from build123d import *

# Parameters (mm, degrees)
SKETCH1_W           = 15
SKETCH1_H           = 30
SKETCH1_R           = 2.5
BOSS_EXTRUDE1_DEPTH = 3
SKETCH2_W           = 15
SKETCH2_H           = 18
SKETCH2_R           = 2.5
BOSS_EXTRUDE2_DEPTH = 3
BOSS_EXTRUDE3_DEPTH = 2


with BuildPart() as part:
    # Sketch1 → Boss-Extrude1 (new body)
    with BuildSketch(Plane.XY):
        Rectangle(SKETCH1_W, SKETCH1_H)
        with Locations((0, 8)):
            Circle(SKETCH1_R, mode=Mode.SUBTRACT)
        with Locations((0, -8)):
            Circle(SKETCH1_R, mode=Mode.SUBTRACT)
    extrude(amount=BOSS_EXTRUDE1_DEPTH)

    # Sketch2 → Boss-Extrude2 (add)
    with BuildSketch(Plane(origin=(0, 15, 0), x_dir=(1, 0, 0), z_dir=(0, 1, 0))):
        with Locations((0, 6)):
            Rectangle(SKETCH2_W, SKETCH2_H)
        with Locations((0, 7.5)):
            Circle(SKETCH2_R, mode=Mode.SUBTRACT)
    extrude(amount=BOSS_EXTRUDE2_DEPTH)

    # Sketch3 → Boss-Extrude3 (add)
    with BuildSketch(Plane(origin=(7.5, 0, 0), x_dir=(0, 0, -1), z_dir=(1, 0, 0))):
        Polygon((15, 15), (0, 0), (0, 15), align=None)
    boss_extrude3 = extrude(amount=-BOSS_EXTRUDE3_DEPTH)

    # Mirror1: Boss-Extrude3 across plane
    add(boss_extrude3.mirror(Plane(origin=(0, 0, 0), x_dir=(0, 0, 1), z_dir=(1, 0, 0))))


solid = part.part
Source: CAD feature listing. Evaluate the final solid. Frame: model axes, mm. A direction names the side the tool comes from. Coordinates: 2 decimals unless noted, no trailing zeros. Loops run counter-clockwise (first coordinate to the right, second up) from the corner with the lowest first, then second, coordinate; pieces in that order, holes last. Notation, with made-up numbers: (-24.5, 43.25) -> (17.5, 43.25) arc R19 cw to (17.5, 63.25) -> close; hole circle Ø5 at (34.25, 89.5). An arc over 180 degrees is marked (long way). Answer in a Markdown table with one row per item. Add a question column.
Q1. Ray query, line 1 along Y through (x, z) = (0, 0.95); line 2 along X through (y, z) = (7, -6.5); line 3 along Z through (x, y) = (0, 16.6). Return the intervals inside material, ascending.
Q2. Section A-A on y = 6. Return the cut outline in (x, z).
Q3. Contact query for flat-ended pins moving along their axis: pin 1 Ø1.5 at (y, z) = (1, -2) entering from +X; pin 2 Ø4 at (x, y) = (0, -8) entering from -Z; pin 3 Ø4.5 at (x, y) = (0.5, 7) entering from -Z; pin 4 Ø5 at (x, y) = (5.5, 10.5) entering from -Z. Output: stop coordinate, or through.
Q4. Section B-B on x = 0. Return the cut outline in (y, z), and give its area (3 significant figures).
Q5. Pull-direction query (Y, two-part tool) for faces 3 (the face through (7, 8, -8)), 4 (the face through (-0.54, -10.44, 1.48)), 5 (the face through (0, 18, -4)); classes: pulls with the +Y half, pulls with the -Y half, needs draft (parallel to the pull), parting line crosses it, or undercut.
Q6. Section D-D on z = 1.25. Return the cut outline in (x, y), and give its area (3 significant figures).
Q7. Section C-C on z = -7.5. Return the cut outline in (x, y).
Q8. Reachability of faces 1 (the face through (-7.5, 9, -4)), 2 (the face through (0, 0, 0)) from +Z, -Z, +X, -X, +Y, -Y: full face, straight path, thin tool, end or side. Return the list, or none.
Computed values:
| question | item | result |
|---|---|---|
| 1 | line 1 | y = -15 to -10.5, -5.5 to 5.5, 10.5 to 18 |
| 1 | line 2 | x = -7.5 to -5.5, 5.5 to 7.5 |
| 1 | line 3 | z = -15 to -10, -5 to 3 |
| 2 | outline | (-7.5, -6) -> (-5.5, -6) -> (-5.5, 0) -> (-1.5, 0) -> (-1.5, 3) -> (-7.5, 3) -> close; (1.5, 0) -> (5.5, 0) -> (5.5, -6) -> (7.5, -6) -> (7.5, 3) -> (1.5, 3) -> close |
| 3 | pin 1 | stops at x = 7.5 |
| 3 | pin 2 | passes through |
| 3 | pin 3 | stops at z = 0 |
| 3 | pin 4 | stops at z = -13 |
| 4 | outline | (-15, 0) -> (-10.5, 0) -> (-10.5, 3) -> (-15, 3) -> close; (-5.5, 0) -> (5.5, 0) -> (5.5, 3) -> (-5.5, 3) -> close; (10.5, 0) -> (15, 0) -> (15, -5) -> (18, -5) -> (18, 3) -> (10.5, 3) -> close; (15, -15) -> (18, -15) -> (18, -10) -> (15, -10) -> close |
| 4 | area | 99.0 mm^2 |
| 5 | face 3 | pulls with the -Y half |
| 5 | face 4 | undercut |
| 5 | face 5 | pulls with the +Y half |
| 6 | outline | (-7.5, -15) -> (7.5, -15) -> (7.5, 18) -> (-7.5, 18) -> close; hole circle Ø5 at (0, -8); hole circle Ø5 at (0, 8) |
| 6 | area | 456 mm^2 |
| 7 | outline | (-7.5, 7.5) -> (-5.5, 7.5) -> (-5.5, 15) -> (-2.5, 15) -> (-2.5, 18) -> (-7.5, 18) -> close; (2.5, 15) -> (5.5, 15) -> (5.5, 7.5) -> (7.5, 7.5) -> (7.5, 18) -> (2.5, 18) -> close |
| 8 | face 1 | +Z, -Z, -X, +Y, -Y |
| 8 | face 2 | -Z, -Y |
